from build123d import *

# Parameters (mm, degrees)
SKETCH1_W           = 42
SKETCH1_H           = 47.5
BOSS_EXTRUDE1_DEPTH = 1
SKETCH2_W           = 15
SKETCH2_H           = 12
SKETCH2_W_2         = 12
SKETCH2_H_2         = 9
CUT_EXTRUDE3_DEPTH  = 25


with BuildPart() as part:
    # Sketch1 → Boss-Extrude1 (new body)
    with BuildSketch(Plane(origin=(0, 0, 0), x_dir=(1, 0, 0), z_dir=(0, 1, 0))):
        Rectangle(SKETCH1_W, SKETCH1_H)
    extrude(amount=BOSS_EXTRUDE1_DEPTH)

    # Sketch2 → Cut-Extrude3 (cut)
    with BuildSketch(Plane(origin=(0, 0, 0), x_dir=(1, 0, 0), z_dir=(0, 1, 0))):
        with Locations((-0.5, -10.75)):
            Rectangle(SKETCH2_W, SKETCH2_H)
        with Locations((1, 9.75)):
            Rectangle(SKETCH2_W_2, SKETCH2_H_2)
    extrude(amount=CUT_EXTRUDE3_DEPTH, mode=Mode.SUBTRACT)


solid = part.part
CAD build for the part. Positions are in the model's coordinates, mm. A direction names the side the tool comes from. Round coordinates to 2 decimals unless told otherwise and drop trailing zeros. Write each loop counter-clockwise with the first axis right and the second up, starting at its lowest first coordinate (ties: lowest second). Pieces come first, ordered by that corner, then holes.
(1) Probe line 1 along Z through (x, y) = (3.5, 0.3); line 2 along X through (y, z) = (0.7, 10); line 3 along X through (y, z) = (0.9, -14). List the from-to ranges inside material, lowest first.
(2) Slice it at A-A, the plane z = 13.5. Write the cut outline in (x, y).
(3) Slice it at D-D, the plane z = -7. Write the cut outline in (x, y), and give its area (3 significant figures).
(4) Slice it at B-B, the plane y = 0.85. Write the cut outline in (x, z).
(5) 3-axis set-ups, long thin cutter, end or side, ignore diameter. For faces 5 (the face through (0.9, 0.5, -5.25)), 6 (the face through (-0.3, 0.5, -23.75)): which of +Z, -Z, +X, -X, +Y, -Y reach the whole face in a straight line?
(6) Slice it at C-C, the plane x = -1.5. Write the cut outline in (y, z), and give its area (3 significant figures).
(7) Mould opens along X. For faces 1 (the face through (7, 0.5, -9.7)), 2 (the face through (21, 0.5, 0.3)), 3 (the face through (0, 1, 0)), 4 (the face through (-0.6, 0.5, 16.75)) say: pulls with the +X half, pulls with the -X half, needs draft (parallel to the pull), parting line crosses it, or undercut.
From the geometry:
1. line 1: z = -23.75 to -14.25, -5.25 to 4.75, 16.75 to 23.75
1. line 2: x = -21 to -8, 7 to 21
1. line 3: x = -21 to -5, 7 to 21
2. outline: (-21, 0) - (-8, 0) - (-8, 1) - (-21, 1) - close; (7, 0) - (21, 0) - (21, 1) - (7, 1) - close
3. outline: (-21, 0) - (-5, 0) - (-5, 1) - (-21, 1) - close; (7, 0) - (21, 0) - (21, 1) - (7, 1) - close
3. area: 30.0 mm2
4. outline: (-21, -23.75) - (21, -23.75) - (21, 23.75) - (-21, 23.75) - close; hole (-8, 4.75) - (7, 4.75) - (7, 16.75) - (-8, 16.75) - close; hole (-5, -14.25) - (7, -14.25) - (7, -5.25) - (-5, -5.25) - close
5. face 5: +Y, -Y
5. face 6: -Z, +X, -X, +Y, -Y
6. outline: (0, -23.75) - (1, -23.75) - (1, -14.25) - (0, -14.25) - close; (0, -5.25) - (1, -5.25) - (1, 4.75) - (0, 4.75) - close; (0, 16.75) - (1, 16.75) - (1, 23.75) - (0, 23.75) - close
6. area: 26.5 mm2
7. face 1: undercut
7. face 2: pulls with the +X half
7. face 3: needs draft
7. face 4: undercut
